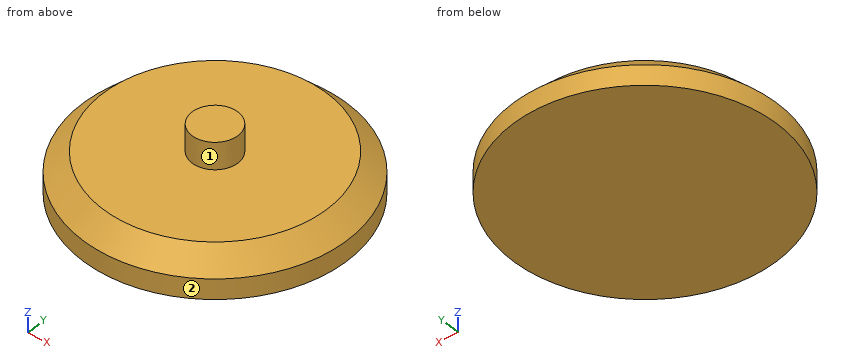
from build123d import *

# Parameters (mm, degrees)
F0_R     = 0.85
F1_DEPTH = 1
F0_R_2   = 4.9
F2_DEPTH = 1.5
F3_SIZE  = 0.75


with BuildPart() as f1:
    # F0 (on Top) → F1 (new body)
    with BuildSketch(Plane.XY):
        Circle(F0_R)
    extrude(amount=F1_DEPTH)

    # F0 (on Top) → F2 (join)
    with BuildSketch(Plane.XY):
        Circle(F0_R_2)
        Circle(F0_R, mode=Mode.SUBTRACT)
        Circle(F0_R)
    extrude(amount=-F2_DEPTH)

    # F3
    f3_edges = [f1.edges().sort_by_distance(p)[0] for p in [
        (-4.9, 0, 0),
    ]]
    chamfer(f3_edges, length=F3_SIZE)


solid = f1.part
Can you work these out from the model? Positions are in its coordinate system, mm. Face numbers are marked on the shaded views. A direction names the side the tool comes from. Give positions to 0.01 mm unless a question says otherwise; leave off trailing zeros. Write each loop counter-clockwise with the first axis right and the second up, starting at its lowest first coordinate (ties: lowest second). Pieces come first, ordered by that corner, then holes. Notation, with made-up numbers: (-3.75, 6) -> (22.25, 6) arc R19 cw to (22.25, 11) -> close; hole circle Ø1 at (-7, 24.5). An arc over 180 degrees is marked (long way). Answer as a JSON object with one key per item and string values. Group by question number.
Item 1: Suppose I cut it at C-C (z = -0.15). Please give me the cut outline in (x, y).
Item 2: Please list where these lines run through material, in increasing order: line 1 (Z direction, x = 0.5, y = 2.5); line 2 (Y direction, x = 0, z = 0.15); line 3 (X direction, y = 4, z = -0.3). Write a range as [from, to].
Item 3: For the marked faces 1 and 2, which set-ups out of +Z, -Z, +X, -X, +Y, -Y let a thin tool reach every point of the face, with its end or its side?
Item 4: Suppose I cut it at A-A (y = 0). Please give me the cut outline in (x, z).
Findings:
{
 "1": {"outline": "circle Ø8.6 at (0, 0)"},
 "2": {"line 1": "z = [-1.5, 0]", "line 2": "y = [-0.85, 0.85]", "line 3": "x = [-1.95, 1.95]"},
 "3": {"face 1": "+Z", "face 2": "+Z, -Z"},
 "4": {"outline": "(-4.9, -1.5) -> (4.9, -1.5) -> (4.9, -0.75) -> (4.15, 0) -> (0.85, 0) -> (0.85, 1) -> (-0.85, 1) -> (-0.85, 0) -> (-4.15, 0) -> (-4.9, -0.75) -> close"}
}
